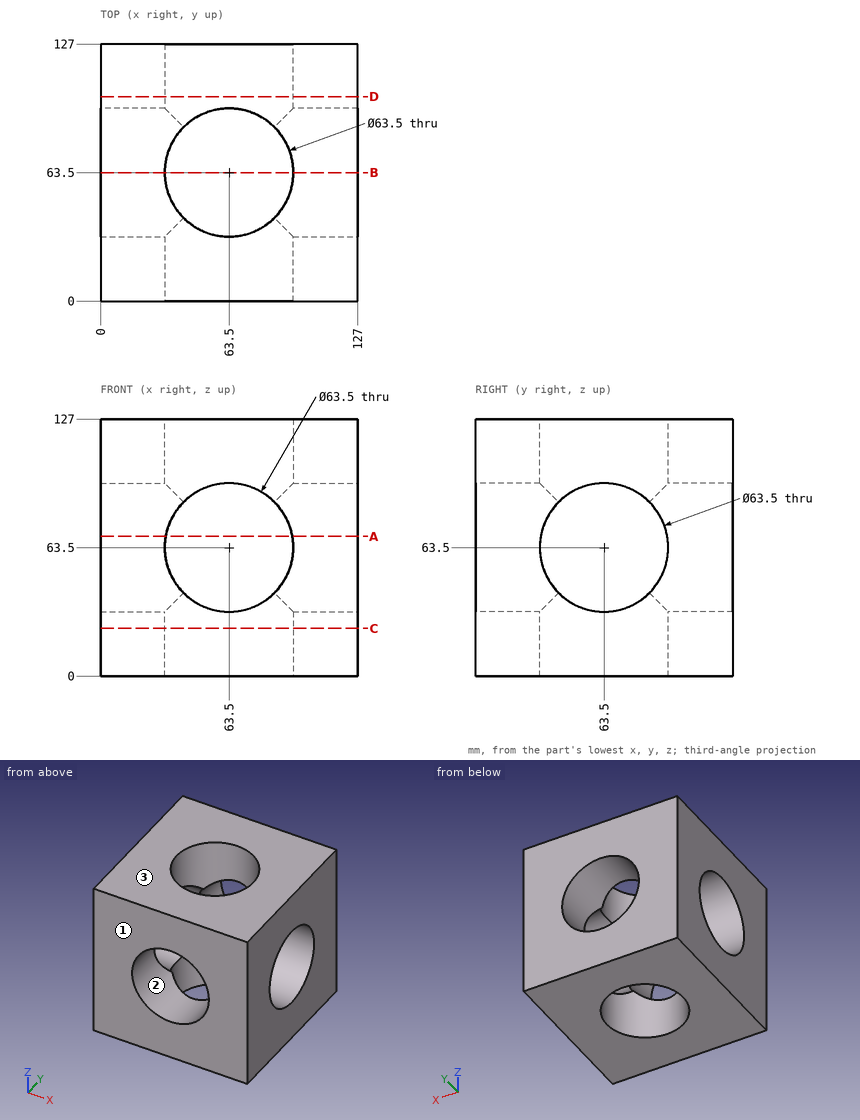
Check sheet for the drawn part. Datum: minimum x, y, z corner. Units: mm. Give positions to 0.01 mm unless a question says otherwise; leave off trailing zeros. Order: outer loops, then holes, each group sorted by start corner. A loop starts at its lowest first (then second) coordinate and runs counter-clockwise, first axis right, second up. Notation, with made-up numbers: (-33.5, 37.25) -> (-9.5, 37.25) arc R14 cw to (-9.5, 47.25) -> close; hole circle Ø9 at (-4, -39). An arc over 180 degrees is marked (long way). One line per item, written item: value.
(1) Sectioned sample at C-C on z = 23.5. Record the cut outline in (x, y), then the cut area to 3 significant figures.
Final values:
outline: (0, 0) -> (127, 0) -> (127, 127) -> (0, 127) -> close; hole circle Ø63.5 at (63.5, 63.5)
area: 13,000 mm^2
(2) Sectioned sample at B-B on y = 63.5. Record the cut outline in (x, z).
Final values:
outline: (0, 0) -> (31.75, 0) -> (31.75, 31.75) -> (0, 31.75) -> close; (0, 95.25) -> (31.75, 95.25) -> (31.75, 127) -> (0, 127) -> close; (95.25, 0) -> (127, 0) -> (127, 31.75) -> (95.25, 31.75) -> close; (95.25, 95.25) -> (127, 95.25) -> (127, 127) -> (95.25, 127) -> close
(3) Scan line: line 1 along Y through (x, z) = (63.5, 115). Record every from-to range of solid material in increasing order. Write a range as [from, to].
Final values:
line 1: [0, 31.75], [95.25, 127]
(4) Sectioned sample at A-A on z = 69. Record the cut outline in (x, y), then the cut area to 3 significant figures.
Final values:
outline: (0, 0) -> (32.23, 0) -> (32.23, 32.23) -> (0, 32.23) -> close; (0, 94.77) -> (32.23, 94.77) -> (32.23, 127) -> (0, 127) -> close; (94.77, 0) -> (127, 0) -> (127, 32.23) -> (94.77, 32.23) -> close; (94.77, 94.77) -> (127, 94.77) -> (127, 127) -> (94.77, 127) -> close
area: 4,160 mm^2
(5) Draft check along Z on the marked faces 1, 2 and 3. Enter one of: pulls with the +Z half, pulls with the -Z half, needs draft (parallel to the pull), parting line crosses it, or undercut.
Final values:
face 1: needs draft
face 2: undercut
face 3: pulls with the +Z half
(6) Gauge pin test, flat end, axial feed: pin 1 (1.5 mm diameter, centred on x = 80.5, z = 38, fed in from -Y). Record the tip position at first contact, or that the pin passes through.
Final values:
pin 1: through
